Build history of the part. All positions in model axes, mm. Face numbers are marked on the shaded views. A direction names the side the tool comes from. Coordinates: 2 decimals unless noted, no trailing zeros. Write each loop counter-clockwise with the first axis right and the second up, starting at its lowest first coordinate (ties: lowest second). Pieces come first, ordered by that corner, then holes.
from build123d import *

# Parameters (mm, degrees)
SKETCH1_W           = 330.2
SKETCH1_H           = 127
BOSS_EXTRUDE1_DEPTH = 12.7
CUT_EXTRUDE1_DEPTH  = 3.556
SKETCH3_W           = 25.4
SKETCH3_H           = 12.7
BOSS_EXTRUDE2_DEPTH = 12.7
SKETCH4_R           = 3.2385
CUT_EXTRUDE2_DEPTH  = 25.4
SKETCH5_R           = 5.08
CUT_EXTRUDE3_DEPTH  = 6.35
SKETCH6_R           = 2.5527
CUT_EXTRUDE4_DEPTH  = 25.4


with BuildPart() as part:
    # Sketch1 → Boss-Extrude1 (new body)
    with BuildSketch(Plane(origin=(0, 0, 0), x_dir=(1, 0, 0), z_dir=(0, 1, 0))):
        Rectangle(SKETCH1_W, SKETCH1_H)
    extrude(amount=BOSS_EXTRUDE1_DEPTH)

    # Sketch2 → Cut-Extrude1 (cut)
    with BuildSketch(Plane(origin=(0, 12.7, 0), x_dir=(1, 0, 0), z_dir=(0, 1, 0))):
        with BuildLine():
            Line((-89.555550869, 44.45), (89.555550869, 44.45))
            ThreePointArc((89.555550869, 44.45), (95.848789674, 38.947139505), (91.234685107, 31.976030029))
            Line((91.234685107, 31.976030029), (6.256412404, 8.675797038))
            ThreePointArc((6.256412404, 8.675797038), (0, 7.833614774), (-6.256412404, 8.675797038))
            Line((-6.256412404, 8.675797038), (-91.234685107, 31.976030029))
            ThreePointArc((-91.234685107, 31.976030029), (-95.848789674, 38.947139505), (-89.555550869, 44.45))
        make_face()
        with BuildLine():
            Line((-152.4, 26.105568393), (-152.4, -25.353616872))
            ThreePointArc((-152.4, -25.353616872), (-149.556629033, -31.098337724), (-143.26451887, -32.321418189))
            Line((-143.26451887, -32.321418189), (-49.42612935, -6.591825556))
            ThreePointArc((-49.42612935, -6.591825556), (-44.111657731, 0.375975761), (-49.42612935, 7.343777077))
            Line((-49.42612935, 7.343777077), (-143.26451887, 33.07336971))
            ThreePointArc((-143.26451887, 33.07336971), (-149.556629033, 31.850289245), (-152.4, 26.105568393))
        make_face()
        with BuildLine():
            Line((-92.297993035, -44.45), (92.297993035, -44.45))
            ThreePointArc((92.297993035, -44.45), (98.59123184, -38.947139505), (93.977127273, -31.976030029))
            Line((93.977127273, -31.976030029), (6.716536951, -8.050007285))
            ThreePointArc((6.716536951, -8.050007285), (0, -7.145887171), (-6.716536951, -8.050007285))
            Line((-6.716536951, -8.050007285), (-93.977127273, -31.976030029))
            ThreePointArc((-93.977127273, -31.976030029), (-98.59123184, -38.947139505), (-92.297993035, -44.45))
        make_face()
        with BuildLine():
            Line((146.05, 25.51164), (146.05, -24.759688479))
            ThreePointArc((146.05, -24.759688479), (143.550973746, -29.808698402), (138.020865762, -30.88365845))
            Line((138.020865762, -30.88365845), (46.348592305, -5.747994211))
            ThreePointArc((46.348592305, -5.747994211), (41.677726543, 0.375975761), (46.348592305, 6.499945732))
            Line((46.348592305, 6.499945732), (138.020865762, 31.635609971))
            ThreePointArc((138.020865762, 31.635609971), (143.550973746, 30.560649923), (146.05, 25.51164))
        make_face()
    cut_extrude1 = extrude(amount=-CUT_EXTRUDE1_DEPTH, mode=Mode.SUBTRACT)

    # Sketch3 → Boss-Extrude2 (add)
    with BuildSketch(Plane.XZ):
        with Locations((-101.6, 69.85)):
            Rectangle(SKETCH3_W, SKETCH3_H)
        with Locations((-152.4, 69.85)):
            Rectangle(SKETCH3_W, SKETCH3_H)
        with Locations((-50.8, 69.85)):
            Rectangle(SKETCH3_W, SKETCH3_H)
        with Locations((0, 69.85)):
            Rectangle(SKETCH3_W, SKETCH3_H)
        with Locations((50.8, 69.85)):
            Rectangle(SKETCH3_W, SKETCH3_H)
        with Locations((101.6, 69.85)):
            Rectangle(SKETCH3_W, SKETCH3_H)
        with Locations((152.4, 69.85)):
            Rectangle(SKETCH3_W, SKETCH3_H)
        with Locations((-101.6, -69.85)):
            Rectangle(SKETCH3_W, SKETCH3_H)
        with Locations((-50.8, -69.85)):
            Rectangle(SKETCH3_W, SKETCH3_H)
        with Locations((0, -69.85)):
            Rectangle(SKETCH3_W, SKETCH3_H)
        with Locations((50.8, -69.85)):
            Rectangle(SKETCH3_W, SKETCH3_H)
        with Locations((101.6, -69.85)):
            Rectangle(SKETCH3_W, SKETCH3_H)
        with Locations((152.4, -69.85)):
            Rectangle(SKETCH3_W, SKETCH3_H)
        with Locations((-152.4, -69.85)):
            Rectangle(SKETCH3_W, SKETCH3_H)
    extrude(amount=-BOSS_EXTRUDE2_DEPTH)

    # Sketch4 → Cut-Extrude2 (cut)
    with BuildSketch(Plane(origin=(0, 12.7, 0), x_dir=(1, 0, 0), z_dir=(0, 1, 0))):
        with Locations((-152.4, 69.85)):
            Circle(SKETCH4_R)
        with Locations((-101.6, 69.85)):
            Circle(SKETCH4_R)
        with Locations((-50.8, 69.85)):
            Circle(SKETCH4_R)
        with Locations((0, 69.85)):
            Circle(SKETCH4_R)
        with Locations((50.8, 69.85)):
            Circle(SKETCH4_R)
        with Locations((101.6, 69.85)):
            Circle(SKETCH4_R)
        with Locations((152.4, 69.85)):
            Circle(SKETCH4_R)
        with Locations((-101.6, -69.85)):
            Circle(SKETCH4_R)
        with Locations((-50.8, -69.85)):
            Circle(SKETCH4_R)
        with Locations((0, -69.85)):
            Circle(SKETCH4_R)
        with Locations((50.8, -69.85)):
            Circle(SKETCH4_R)
        with Locations((101.6, -69.85)):
            Circle(SKETCH4_R)
        with Locations((152.4, -69.85)):
            Circle(SKETCH4_R)
        with Locations((-152.4, -69.85)):
            Circle(SKETCH4_R)
    extrude(amount=-CUT_EXTRUDE2_DEPTH, mode=Mode.SUBTRACT)

    # Sketch5 → Cut-Extrude3 (cut)
    with BuildSketch(Plane(origin=(0, 12.7, 0), x_dir=(1, 0, 0), z_dir=(0, 1, 0))):
        with Locations((-152.4, 69.85)):
            Circle(SKETCH5_R)
        with Locations((-101.6, 69.85)):
            Circle(SKETCH5_R)
        with Locations((-50.8, 69.85)):
            Circle(SKETCH5_R)
        with Locations((0, 69.85)):
            Circle(SKETCH5_R)
        with Locations((50.8, 69.85)):
            Circle(SKETCH5_R)
        with Locations((101.6, 69.85)):
            Circle(SKETCH5_R)
        with Locations((152.4, 69.85)):
            Circle(SKETCH5_R)
        with Locations((-101.6, -69.85)):
            Circle(SKETCH5_R)
        with Locations((-50.8, -69.85)):
            Circle(SKETCH5_R)
        with Locations((0, -69.85)):
            Circle(SKETCH5_R)
        with Locations((50.8, -69.85)):
            Circle(SKETCH5_R)
        with Locations((101.6, -69.85)):
            Circle(SKETCH5_R)
        with Locations((152.4, -69.85)):
            Circle(SKETCH5_R)
        with Locations((-152.4, -69.85)):
            Circle(SKETCH5_R)
    extrude(amount=-CUT_EXTRUDE3_DEPTH, mode=Mode.SUBTRACT)

    # Sketch6 → Cut-Extrude4 (cut)
    with BuildSketch(Plane.XY.offset(63.5)):
        with Locations((-127, 6.35)):
            Circle(SKETCH6_R)
        with Locations((-76.2, 6.35)):
            Circle(SKETCH6_R)
        with Locations((-25.4, 6.35)):
            Circle(SKETCH6_R)
        with Locations((25.4, 6.35)):
            Circle(SKETCH6_R)
        with Locations((76.2, 6.35)):
            Circle(SKETCH6_R)
        with Locations((127, 6.35)):
            Circle(SKETCH6_R)
    cut_extrude4 = extrude(amount=-CUT_EXTRUDE4_DEPTH, mode=Mode.SUBTRACT)

    # Mirror1: Cut-Extrude4 across plane
    add(cut_extrude4.mirror(Plane(origin=(0, 0, 0), x_dir=(1, 0, 0), z_dir=(0, 0, -1))), mode=Mode.SUBTRACT)

    # Mirror2: Cut-Extrude1 across plane
    add(cut_extrude1.mirror(Plane.ZX.offset(6.35)), mode=Mode.SUBTRACT)


solid = part.part
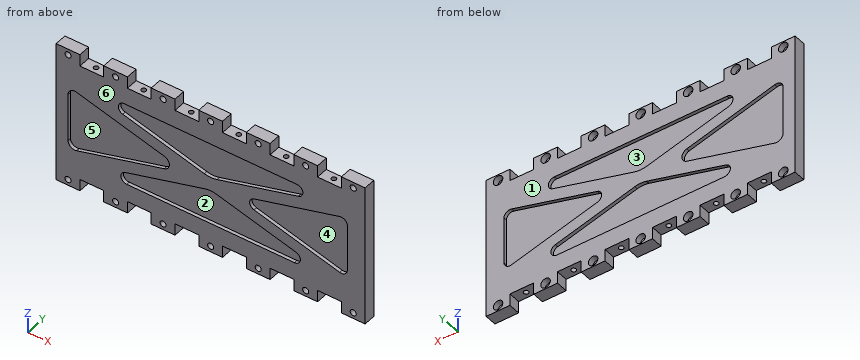
(1) Probe L1, parallel to Z at x = 50.8, y = 5; L2, parallel to Y at x = 76.2, z = 47.25; L3, parallel to Z at x = -11, y = 3. List the from-to ranges inside material, lowest first.
(2) Flat gauge pins, fed straight in: P1, Ø3, axis at x = -51.5, z = -68, coming from the +Y side; P2, Ø3, axis at x = 127, y = 6.35, coming from the +Z side; P3, Ø4, axis at x = -50.8, z = 69.85, coming from the -Y side; P4, Ø4, axis at x = -127, y = 6.35, coming from the -Z side. Where does each tip first touch, or does it go through?
(3) Two-plate mould, pull along X, no slides. Class the marked faces 4, 5 and 6: pulls with the +X half, pulls with the -X half, needs draft (parallel to the pull), parting line crosses it, or undercut.
(4) Slice it at A-A, the plane z = 52. List the corners of the cut face in (x, y), and give its area (3 significant figures).
(5) Slice it at B-B, the plane x = -133. List the corners of the cut face in (y, z).
(6) Slice it at C-C, the plane z = -69.85. Give the number of separate pieces and of enclosed holes in the cut face, and give its area (3 significant figures).
(7) 3-axis set-ups, long thin cutter, end or side, ignore diameter. For the marked faces 1, 2 and 3: which of +Z, -Z, +X, -X, +Y, -Y reach the whole face in a straight line?
Results:
1. L1: z = -76.2 to -73.09, -66.61 to 66.61, 73.09 to 76.2
1. L2: y = 0 to 3.8, 8.9 to 12.7
1. L3: z = -76.2 to -44.45, -9.98 to 9.22, 44.45 to 76.2
2. P1: stops at y = 6.35
2. P2: stops at z = 38.1
2. P3: passes through
2. P4: stops at z = -38.1
3. face 4: undercut
3. face 5: undercut
3. face 6: needs draft
4. outline: (-165.1, 0) - (165.1, 0) - (165.1, 12.7) - (-165.1, 12.7) - close; hole circle Ø5.11 at (-127, 6.35); hole circle Ø5.11 at (-76.2, 6.35); hole circle Ø5.11 at (-25.4, 6.35); hole circle Ø5.11 at (25.4, 6.35); hole circle Ø5.11 at (76.2, 6.35); hole circle Ø5.11 at (127, 6.35)
4. area: 4,070 mm2
5. outline: (0, -63.5) - (12.7, -63.5) - (12.7, -30.26) - (9.14, -30.26) - (9.14, 29.51) - (12.7, 29.51) - (12.7, 63.5) - (0, 63.5) - (0, 29.51) - (3.56, 29.51) - (3.56, -30.26) - (0, -30.26) - close
6. separate pieces: 14
6. enclosed holes: 0
6. area: 1,520 mm2
7. face 1: +Z, -Z, +X, -X, +Y
7. face 2: -Y
7. face 3: +Y
